Could you check a few things on this drawing? It's one solid part, dimensions in mm from its lowest x, y, z. Give positions to 0.01 mm unless a question says otherwise; leave off trailing zeros. Order: outer loops, then holes, each group sorted by start corner. A loop starts at its lowest first (then second) coordinate and runs counter-clockwise, first axis right, second up. Notation, with made-up numbers: (49, 65.5) - (86, 65.5) arc R24 cw to (86, 104.5) - close; hole circle Ø8 at (52, 35). An arc over 180 degrees is marked (long way). One line per question, with ' | ' between items. Start each with the question number.
1. Imagine slicing it at A-A (x = 92). Please give me the cut outline in (y, z) (1 decimal).
2. For P1, Ø1.6, axis at x = 211.5, y = 2, coming from the -Z side; P2, Ø1.6, axis at y = 1, z = 80.5, coming from the -X side; P3, Ø1.6, axis at y = 1.5, z = 236, coming from the +X side, each with a flat end and sliding along its axis, tell me the tip position at first contact or that it passes through.
3. Imagine slicing it at C-C (y = 1.35). Give the number of separate pieces and of enclosed holes in the cut face, and give its area (3 significant figures).
4. I need wall thicknesses on probe 1 along Z at (x, y) = (78, 2.3); probe 2 along X at (y, z) = (1.5, 131.5); probe 3 along X at (y, z) = (0.45, 207). Which ranges of each line are inside material? Lowest first, please. Write a range as from..to.
5. Imagine slicing it at B-B (z = 140). Please give me the cut outline in (x, y) (1 decimal).
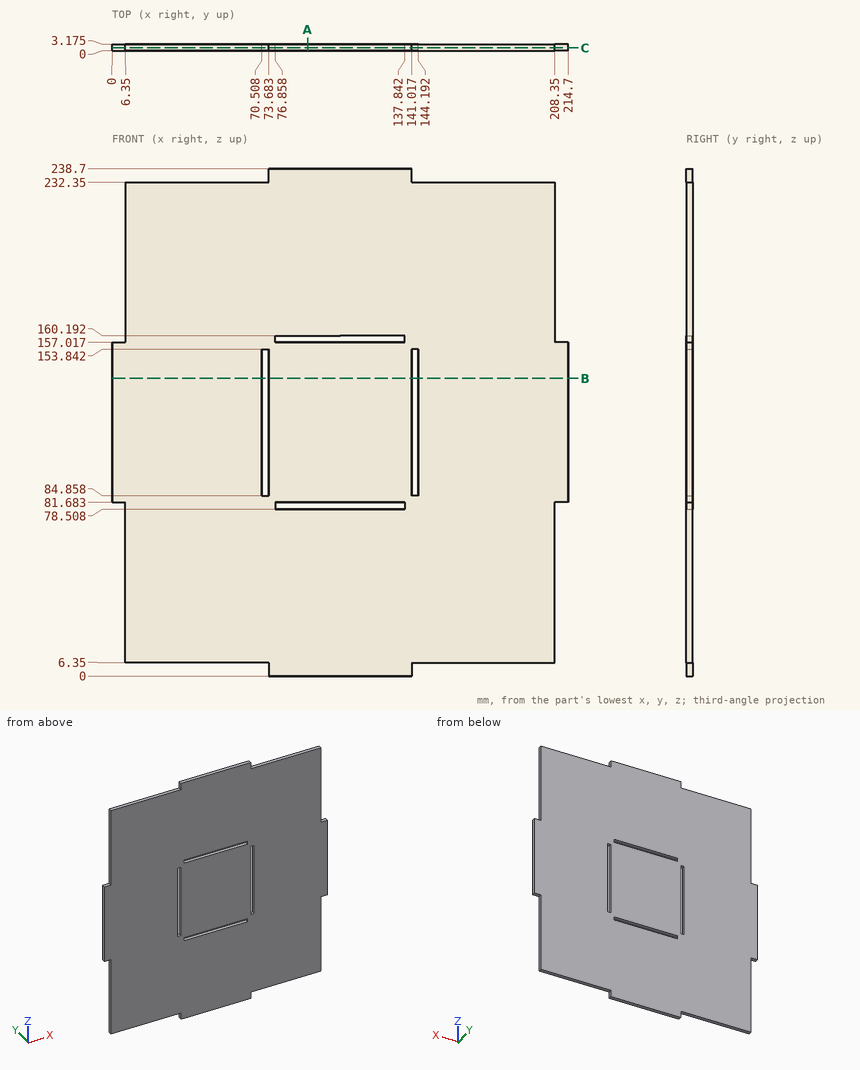
Results found:
1) outline: (0, 0) - (3.2, 0) - (3.2, 78.5) - (0, 78.5) - close; (0, 81.7) - (3.2, 81.7) - (3.2, 157) - (0, 157) - close; (0, 160.2) - (3.2, 160.2) - (3.2, 238.7) - (0, 238.7) - close
2) P1: stops at z = 81.68 | P2: stops at x = 6.35 | P3: stops at x = 141.02
3) separate pieces: 1 | enclosed holes: 4 | area: 46,600 mm2
4) probe 1: z = 0..78.51, 81.68..157.02, 160.19..238.7 | probe 2: x = 0..70.51, 73.68..141.02, 144.19..214.7 | probe 3: x = 6.35..208.35
5) outline: (0, 0) - (70.5, 0) - (70.5, 3.2) - (0, 3.2) - close; (73.7, 0) - (141, 0) - (141, 3.2) - (73.7, 3.2) - close; (144.2, 0) - (214.7, 0) - (214.7, 3.2) - (144.2, 3.2) - close
